Autodesk Inventor part; units mm, degrees
ref_plane "YZ Plane" through (0, 0, 0) normal (1, 0, 0) x (0, 1, 0)
ref_plane "XZ Plane" through (0, 0, 0) normal (0, 1, 0) x (-1, 0, 0)
ref_plane "XY Plane" through (0, 0, 0) normal (0, 0, 1) x (1, 0, 0)
sketch "Sketch1" plane through (0, 0, 0) normal (0, 0, 1) x (1, 0, 0)
  circle A0 centre (0, 0) radius 47.625
  dimension "d0" = 95.25
extrude "Extrusion1" add sketch "Sketch1" along normal blind 3.175
sketch "Sketch2" plane through (0, 0, 3.175) normal (0, 0, 1) x (1, 0, 0)
  circle A0 centre (0, 41.91) radius 1.5875
  circle A1 centre (-36.2951, 20.955) radius 1.5875
  circle A2 centre (-36.2951, -20.955) radius 1.5875
  circle A3 centre (0, -41.91) radius 1.5875
  circle A4 centre (36.2951, -20.955) radius 1.5875
  circle A5 centre (36.2951, 20.955) radius 1.5875
  point P0 (0, 0)
  dimension "d3" = 3.175
  dimension "d4" = 41.91
  dimension "d7" = 360
extrude "Extrusion2" cut sketch "Sketch2" against normal blind 3.175
sketch "Sketch3" plane through (0, 0, 3.175) normal (0, 0, 1) x (1, 0, 0)
  circle A0 centre (0, 0) radius 25.4
  dimension "d11" = 50.8
extrude "Extrusion3" cut sketch "Sketch3" against normal blind 3.175
sketch "Sketch4" plane through (0, 0, 3.175) normal (0, 0, 1) x (1, 0, 0)
  circle A0 centre (20.795, 25.8191) radius 3.175
  line L0 (0, 0) -> (0, 9.1169)
  circle A1 centre (-20.795, 25.8191) radius 3.175
  dimension "d14" = 6.35
  dimension "d15" = 25.8191
  dimension "d16" = 20.795
extrude "Extrusion4" cut sketch "Sketch4" against normal blind 25.4
properties part number "aftSealInsideDisc" material "ABS Plastic"
Could you check a few things on this model? Use its own coordinates, in mm. Round coordinates to 2 decimals unless told otherwise and drop trailing zeros. Write each loop counter-clockwise with the first axis right and the second up, starting at its lowest first coordinate (ties: lowest second). Pieces come first, ordered by that corner, then holes. Notation, with made-up numbers: (66.5, -30.5) - (87.5, -30.5) arc R23 cw to (87.5, 2.5) - close; hole circle Ø5 at (46.25, 31.5). An arc over 180 degrees is marked (long way). Put each result on its own line as item: value. Start each with the question number.
(1) I need wall thicknesses on probe 1 along Y at (x, z) = (0, 1) (1 decimal); probe 2 along Y at (x, z) = (37.5, 0.35); probe 3 along X at (y, z) = (1, 3). Which ranges of each line are inside material? Lowest first, please.
(2) I want a section at D-D, the plane y = -41.91. Please give me the cut outline in (x, z) (1 decimal).
(3) Will these pins go through, and if not, where does the flat tip stop? pin 1 (1.5 mm diameter, centred on y = 2, z = 2, fed in from -X); pin 2 (1.5 mm diameter, centred on y = -14, z = 0.5, fed in from +X); pin 3 (5 mm diameter, centred on x = -20.8, y = 25.82, fed in from -Z).
(4) I want a section at A-A, the plane x = 0. Please give me the cut outline in (y, z) (1 decimal).
(5) I want a section at B-B, the plane y = 0. Please give me the cut outline in (x, z) (3 decimals).
(6) Thinking about a two-plate mould opening in Y: for faces 1 (the cylindrical face through (-37.794, 28.979, 1.565)), 2 (the flat face through (20, -20, 3.175)), 3 (the cylindrical face through (36.09, -19.38, 1.61)), which applies, released by +Y, released by -Y, zero draft, split by the parting line, or undercut?
(7) I want a section at C-C, the plane z = 0.7. Give the number of separate pieces and of enclosed holes in the cut face, plus the area to 3 significant figures.
Here are the results:
1. probe 1: y = -47.6 to -43.5, -40.3 to -25.4, 25.4 to 40.3, 43.5 to 47.6
1. probe 2: y = -29.36 to -21.99, -19.92 to 19.92, 21.99 to 29.36
1. probe 3: x = -47.61 to -25.38, 25.38 to 47.61
2. outline: (-22.6, 0) - (-1.6, 0) - (-1.6, 3.2) - (-22.6, 3.2) - close; (1.6, 0) - (22.6, 0) - (22.6, 3.2) - (1.6, 3.2) - close
3. pin 1: stops at x = -47.61
3. pin 2: stops at x = 45.74
3. pin 3: passes through
4. outline: (-47.6, 0) - (-43.5, 0) - (-43.5, 3.2) - (-47.6, 3.2) - close; (-40.3, 0) - (-25.4, 0) - (-25.4, 3.2) - (-40.3, 3.2) - close; (25.4, 0) - (40.3, 0) - (40.3, 3.2) - (25.4, 3.2) - close; (43.5, 0) - (47.6, 0) - (47.6, 3.2) - (43.5, 3.2) - close
5. outline: (-47.625, 0) - (-25.4, 0) - (-25.4, 3.175) - (-47.625, 3.175) - close; (25.4, 0) - (47.625, 0) - (47.625, 3.175) - (25.4, 3.175) - close
6. face 1: split by the parting line
6. face 2: zero draft
6. face 3: undercut
7. separate pieces: 1
7. enclosed holes: 9
7. area: 4,990 mm^2
